```python
from build123d import *

# Parameters (mm, degrees)
SKETCH1_W                = 145
SKETCH1_H                = 110
SKETCH1_R                = 2.25
BOSS_EXTRUDE1_DEPTH      = 2
BOSS_EXTRUDE2_DEPTH      = 55
BOSS_EXTRUDE2_DEPTH_BACK = 55


with BuildPart() as part:
    # Sketch1 → Boss-Extrude1 (new body)
    with BuildSketch(Plane.XY):
        Rectangle(SKETCH1_W, SKETCH1_H)
        with Locations((-68, -47.5)):
            Circle(SKETCH1_R, mode=Mode.SUBTRACT)
        with Locations(Location((68, -47.5, 0), (0, 0, 180))):
            Circle(SKETCH1_R, mode=Mode.SUBTRACT)
        with Locations((68, 47.5)):
            Circle(SKETCH1_R, mode=Mode.SUBTRACT)
        with Locations(Location((-68, 47.5, 0), (0, 0, 180))):
            Circle(SKETCH1_R, mode=Mode.SUBTRACT)
    extrude(amount=BOSS_EXTRUDE1_DEPTH)

    # Sketch3 → Boss-Extrude2 (add, two sides: drawn at the far end of the back side and taken through both)
    with BuildSketch(Plane(origin=(0, 0, 0), x_dir=(1, 0, 0), z_dir=(0, 1, 0)).offset(-BOSS_EXTRUDE2_DEPTH_BACK)):
        Polygon((-72.5, 0), (-72.5, 45), (-47.5, 45), (-47.5, 64), (32.5, 64), (32.5, 40), (72.5, 40), (72.5, 0), align=None)
    extrude(amount=BOSS_EXTRUDE2_DEPTH + BOSS_EXTRUDE2_DEPTH_BACK)


solid = part.part
```
Work out the finished part from the listing and answer in its coordinate system (mm). A direction names the side the tool comes from. Round coordinates to 2 decimals unless told otherwise and drop trailing zeros. Write each loop counter-clockwise with the first axis right and the second up, starting at its lowest first coordinate (ties: lowest second). Pieces come first, ordered by that corner, then holes.
1) Consider probe 1 along Y at (x, z) = (68, 1); probe 2 along Z at (x, y) = (51, -48.5); probe 3 along X at (y, z) = (-42, -49.5). Determine where each line is inside the solid, lowest interval first.
2) A cutting plane is placed at B-B on y = -2. Determine the outline of the cut face in (x, z), and give its area (4 significant figures).
3) Which of the six approach directions +Z, -Z, +X, -X, +Y, -Y give full straight-line access (tool end or side, diameter ignored) to faces 4 (the face through (-72.5, -1, -21)), 5 (the face through (32.5, -1, -52)), 6 (the face through (-68, 47, 0)), 7 (the face through (-60, -1, -45))?
4) Flat-ended cylindrical pins translate along their axes: P1, Ø2, axis at x = 67, y = 47, coming from the +Z side; P2, Ø3.5, axis at x = -68, y = 47.5, coming from the -Z side; P3, Ø6, axis at x = 44, y = -25, coming from the -Z side. Find the tip coordinate at first contact, or state that the pin passes through.
5) A cutting plane is placed at A-A on x = 68. Determine the outline of the cut face in (y, z), and give its area (3 significant figures).
6) A cutting plane is placed at C-C on z = -42.5. Determine the outline of the cut face in (x, y), and give its area (4 significant figures).
7) A cutting plane is placed at D-D on x = -68. Determine the outline of the cut face in (y, z).
8) Determine the mould class of faces 1 (the face through (-68, -48, 0)), 2 (the face through (-47.5, -1, -54)), 3 (the face through (72.5, -1, -19)) for opening direction X: pulls with the +X half, pulls with the -X half, needs draft (parallel to the pull), parting line crosses it, or undercut.
Entries:
1. probe 1: y = -55 to -49.75, -45.25 to 45.25, 49.75 to 55
1. probe 2: z = -40 to 2
1. probe 3: x = -47.5 to 32.5
2. outline: (-72.5, -45) - (-47.5, -45) - (-47.5, -64) - (32.5, -64) - (32.5, -40) - (72.5, -40) - (72.5, 2) - (-72.5, 2) - close
2. area: 8,135 mm2
3. face 4: +Z, -Z, -X, +Y, -Y
3. face 5: -Z, +X, +Y, -Y
3. face 6: +Z
3. face 7: -Z, -X, +Y, -Y
4. P1: stops at z = 0
4. P2: stops at z = -45
4. P3: stops at z = -40
5. outline: (-55, -40) - (55, -40) - (55, 2) - (49.75, 2) - (49.75, 0) - (45.25, 0) - (45.25, 2) - (-45.25, 2) - (-45.25, 0) - (-49.75, 0) - (-49.75, 2) - (-55, 2) - close
5. area: 4,600 mm2
6. outline: (-72.5, -55) - (32.5, -55) - (32.5, 55) - (-72.5, 55) - close
6. area: 11,550 mm2
7. outline: (-55, -45) - (55, -45) - (55, 2) - (49.75, 2) - (49.75, 0) - (45.25, 0) - (45.25, 2) - (-45.25, 2) - (-45.25, 0) - (-49.75, 0) - (-49.75, 2) - (-55, 2) - close
8. face 1: undercut
8. face 2: pulls with the -X half
8. face 3: pulls with the +X half
